```python
from build123d import *

# Parameters (mm, degrees)
EXTRUDE1_DEPTH          = 10.4
SKETCH2_OUTSIDE_W       = 72.756
SKETCH2_OUTSIDE_H       = 74.768
SKETCH2_OUTSIDE_R       = 6.5
CUT_EXTRUDE1_DEPTH      = 15.37857202
CUT_EXTRUDE1_DRAFT      = -60
SKETCH4_R               = 4
CUT_EXTRUDE3_DEPTH      = 15.37857202
SKETCH12_OUTSIDE_W      = 19.484
SKETCH12_OUTSIDE_H      = 21.496
SKETCH12_OUTSIDE_R      = 4.8
CUT_EXTRUDE10_DEPTH     = 2.34
SKETCH15_W              = 0.381
SKETCH15_H              = 7.505553499
CUT_EXTRUDE_THIN2_DEPTH = 1.832
CIRPATTERN1_COUNT       = 6
SKETCH3_OUTSIDE_W       = 67.248
SKETCH3_OUTSIDE_H       = 69.26
SKETCH3_OUTSIDE_R       = 6.5
CUT_EXTRUDE2_DEPTH      = 13.788546959
CUT_EXTRUDE2_DRAFT      = -60


with BuildPart() as part:
    # Sketch1 → Extrude1 (new body)
    with BuildSketch(Plane.XY):
        Polygon((0, 7.505553499), (-6.5, 3.75277675), (-6.5, -3.75277675), (0, -7.505553499), (6.5, -3.75277675), (6.5, 3.75277675), align=None)
    extrude(amount=-EXTRUDE1_DEPTH)


with BuildPart() as cut_extrude1_tool:
    # Sketch2 outside → Cut-Extrude1 (with draft: the straight prism first)
    with BuildSketch(Plane.XY):
        Rectangle(SKETCH2_OUTSIDE_W, SKETCH2_OUTSIDE_H)
        Circle(SKETCH2_OUTSIDE_R, mode=Mode.SUBTRACT)
    extrude(amount=-CUT_EXTRUDE1_DEPTH)
    # Cut-Extrude1: the draft: its side faces are tilted about the plane it starts from
    cut_extrude1_sides = [cut_extrude1_tool.faces().sort_by_distance(p)[0] for p in [
        (0, -37.384, -7.68928601),
        (36.378, 0, -7.68928601),
        (0, 37.384, -7.68928601),
        (-36.378, 0, -7.68928601),
        (-6.5, 0, -7.68928601),
    ]]
    draft(cut_extrude1_sides, Plane.XY, CUT_EXTRUDE1_DRAFT)


with BuildPart() as part_1:
    add(part.part)

    # Cut-Extrude1: cut by cut_extrude1_tool
    add(cut_extrude1_tool.part, mode=Mode.SUBTRACT)

    # Sketch4 → Cut-Extrude3 (cut, through all)
    with BuildSketch(Plane.XY):
        Circle(SKETCH4_R)
    extrude(amount=-CUT_EXTRUDE3_DEPTH, mode=Mode.SUBTRACT)

    # Sketch12 outside → Cut-Extrude10 (cut)
    with BuildSketch(Plane(origin=(0, 0, -10.4), x_dir=(-1, 0, 0), z_dir=(0, 0, -1))):
        Rectangle(SKETCH12_OUTSIDE_W, SKETCH12_OUTSIDE_H)
        Circle(SKETCH12_OUTSIDE_R, mode=Mode.SUBTRACT)
    extrude(amount=-CUT_EXTRUDE10_DEPTH, mode=Mode.SUBTRACT)

    # Sketch15 → Cut-Extrude-Thin2 (cut)
    with BuildSketch(Plane(origin=(0, 0, -10.4), x_dir=(-1, 0, 0), z_dir=(0, 0, -1))):
        with Locations((0, -3.75277675)):
            Rectangle(SKETCH15_W, SKETCH15_H)
    cut_extrude_thin2 = extrude(amount=-CUT_EXTRUDE_THIN2_DEPTH, mode=Mode.SUBTRACT)

    # CirPattern1: Cut-Extrude-Thin2 ×6 about axis
    cirpattern1_axis = Axis((0, 0, 0), (0, 0, 1))
    for i in range(1, CIRPATTERN1_COUNT):
        add(cut_extrude_thin2.rotate(cirpattern1_axis, i * 360 / CIRPATTERN1_COUNT), mode=Mode.SUBTRACT)


with BuildPart() as cut_extrude2_tool:
    # Sketch3 outside → Cut-Extrude2 (with draft: the straight prism first)
    with BuildSketch(Plane(origin=(0, 0, -8.06), x_dir=(-1, 0, 0), z_dir=(0, 0, -1))):
        Rectangle(SKETCH3_OUTSIDE_W, SKETCH3_OUTSIDE_H)
        Circle(SKETCH3_OUTSIDE_R, mode=Mode.SUBTRACT)
    extrude(amount=-CUT_EXTRUDE2_DEPTH)
    # Cut-Extrude2: the draft: its side faces are tilted about the plane it starts from
    cut_extrude2_sides = [cut_extrude2_tool.faces().sort_by_distance(p)[0] for p in [
        (0, -34.63, -1.16572652),
        (-33.624, 0, -1.16572652),
        (0, 34.63, -1.16572652),
        (33.624, 0, -1.16572652),
        (6.5, 0, -1.16572652),
    ]]
    draft(cut_extrude2_sides, Plane(origin=(0, 0, -8.06), x_dir=(-1, 0, 0), z_dir=(0, 0, -1)), CUT_EXTRUDE2_DRAFT)


with BuildPart() as part_2:
    add(part_1.part)

    # Cut-Extrude2: cut by cut_extrude2_tool
    add(cut_extrude2_tool.part, mode=Mode.SUBTRACT)


solid = part_2.part
```
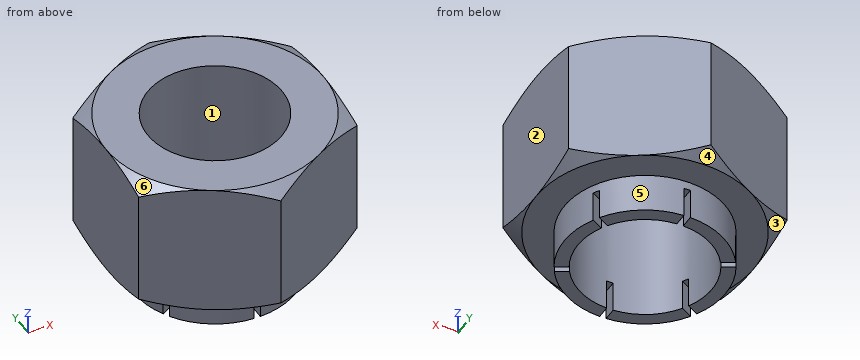
For this review, take the finished solid that the model builds, in its own axes (mm). Face numbers are marked on the shaded views. A direction names the side the tool comes from. Round coordinates to 2 decimals unless told otherwise and drop trailing zeros. Write each loop counter-clockwise with the first axis right and the second up, starting at its lowest first coordinate (ties: lowest second). Pieces come first, ordered by that corner, then holes. Notation, with made-up numbers: (-11, -14) -> (48, -14) arc R16 ccw to (48, 7) -> close; hole circle Ø10 at (83.25, -20). An arc over 180 degrees is marked (long way). Use one line per item in the form item = value.
Q1. Machinability: for the marked faces 5 and 6, which of the approach directions +Z, -Z, +X, -X, +Y, -Y give a long, thin tool a straight path to every point of the face, cutting with its end or side? Answer none if there is none.
Resolved:
face_5 = -Z
face_6 = +Z, -X, -Y
Q2. To check wall thickness, follow probe 1 along Y at (x, z) = (-0.5, -9.5); probe 2 along Y at (x, z) = (1.75, -4.75); probe 3 along X at (y, z) = (0.5, -6.5). State the ranges of each line that lie inside material, in increasing order. Write a range as from..to.
Resolved:
probe_1 = -4.77..-3.97, 3.97..4.77
probe_2 = -6.5..-3.6, 3.6..6.5
probe_3 = -6.5..-3.97, 3.97..6.5
Q3. Consider section A-A (z = -5). State the section outline as (x, y) points.
Resolved:
outline = (-6.5, -3.75) -> (0, -7.51) -> (6.5, -3.75) -> (6.5, 3.75) -> (0, 7.51) -> (-6.5, 3.75) -> close; hole circle Ø8 at (0, 0)
Q4. Consider section B-B (z = -8.25). State the section outline as (x, y) points, then the cut area to 3 significant figures.
Resolved:
outline = circle Ø9.6 at (0, 0); hole circle Ø8 at (0, 0)
area = 22.1 mm²
Q5. Clearance check with flat-ended pins moving along their axes: pin 1 Ø0.6 at (y, z) = (-4, -10) entering from +X; pin 2 Ø2 at (x, y) = (-5, 5.5) entering from -Z; pin 3 Ø0.6 at (y, z) = (-4.5, -9.5) entering from -X. State where each tip first meets the part, or that it passes through.
Resolved:
pin_1 = 3.06
pin_2 = -8.06
pin_3 = -2.32
Q6. The part is to be moulded in two halves that separate along X. For the marked faces 1, 2, 3 and 4, say which applies: released by +X, released by -X, zero draft, split by the parting line, or undercut.
Resolved:
face_1 = undercut
face_2 = released by +X
face_3 = released by -X
face_4 = split by the parting line
